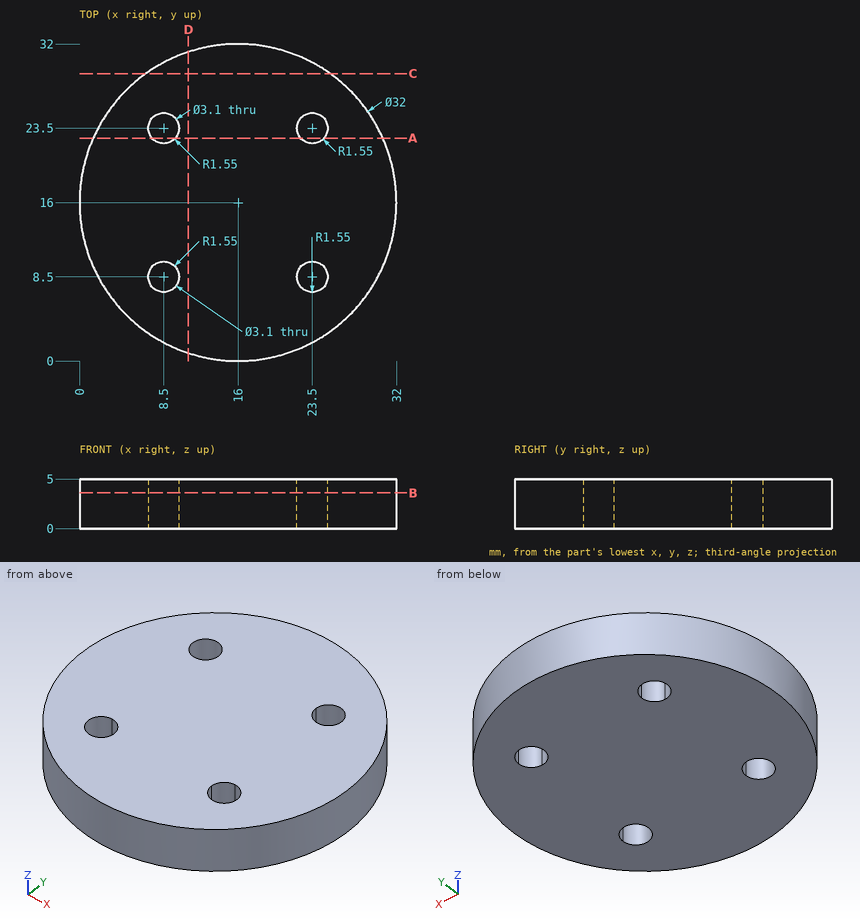
Can you work these out from the drawing? Everything is in mm from the part's minimum corner. Give positions to 0.01 mm unless a question says otherwise; leave off trailing zeros. Loops run counter-clockwise (first coordinate to the right, second up) from the corner with the lowest first, then second, coordinate; pieces in that order, holes last. Notation, with made-up numbers: (61, -34) -> (101, -34) arc R30 cw to (101, -7) -> close; hole circle Ø10 at (-22.75, -19.5). An arc over 180 degrees is marked (long way). Return JSON: item names as keys, results as strings.
Q1. I want a section at B-B, the plane z = 3.6. List the corners of the cut face in (x, y) for me, then the cut area to 3 significant figures.
Checks:
{"outline": "circle Ø32 at (16, 16); hole circle Ø3.1 at (8.5, 8.5); hole circle Ø3.1 at (8.5, 23.5); hole circle Ø3.1 at (23.5, 8.5); hole circle Ø3.1 at (23.5, 23.5)", "area": "774 mm2"}
Q2. I want a section at C-C, the plane y = 29. List the corners of the cut face in (x, z) for me, then the cut area to 3 significant figures.
Checks:
{"outline": "(6.67, 0) -> (25.33, 0) -> (25.33, 5) -> (6.67, 5) -> close", "area": "93.3 mm2"}
Q3. I want a section at A-A, the plane y = 22.5. List the corners of the cut face in (x, z) for me, then the cut area to 3 significant figures.
Checks:
{"outline": "(1.38, 0) -> (7.32, 0) -> (7.32, 5) -> (1.38, 5) -> close; (9.68, 0) -> (22.32, 0) -> (22.32, 5) -> (9.68, 5) -> close; (24.68, 0) -> (30.62, 0) -> (30.62, 5) -> (24.68, 5) -> close", "area": "123 mm2"}
Q4. I need wall thicknesses on probe 1 along X at (y, z) = (8.5, 2.1); probe 2 along X at (y, z) = (8, 0.75). Which ranges of each line are inside material? Lowest first, please.
Checks:
{"probe 1": "x = 1.87 to 6.95, 10.05 to 21.95, 25.05 to 30.13", "probe 2": "x = 2.14 to 7.03, 9.97 to 22.03, 24.97 to 29.86"}
Q5. I want a section at D-D, the plane x = 11. List the corners of the cut face in (y, z) for me.
Checks:
{"outline": "(0.8, 0) -> (31.2, 0) -> (31.2, 5) -> (0.8, 5) -> close"}
Q6. For pin 1 Ø2.5 at (x, y) = (8.5, 8.5) entering from -Z; pin 2 Ø1.5 at (x, z) = (14, 2.5) entering from +Y, each with a flat end and sliding along its axis, tell me the tip position at first contact or that it passes through.
Checks:
{"pin 1": "passes through", "pin 2": "stops at y = 31.95"}
